```python
from build123d import *

# Parameters (mm, degrees)
SKETCH1_R           = 45
SKETCH1_R_2         = 25
BOSS_EXTRUDE1_DEPTH = 3


with BuildPart() as part:
    # Sketch1 → Boss-Extrude1 (new body)
    with BuildSketch(Plane(origin=(0, 0, 0), x_dir=(1, 0, 0), z_dir=(0, 1, 0))):
        with Locations(Location((0, 0, 0), (0, 0, 270))):
            Circle(SKETCH1_R)
        with Locations(Location((0, 0, 0), (0, 0, 270))):
            Circle(SKETCH1_R_2, mode=Mode.SUBTRACT)
        Polygon((-7.346, 39.573965988), (7.346, 39.573965988), (5.573, 29.223349757), (-5.573, 29.223349757), align=None, mode=Mode.SUBTRACT)
        Polygon((9.785315303, 28.094663273), (13.425160378, 37.945059874), (26.14880561, 30.599059874), (19.438034454, 22.521663273), align=None, mode=Mode.SUBTRACT)
        Polygon((22.521663273, 19.438034454), (30.599059874, 26.14880561), (37.945059874, 13.425160378), (28.094663273, 9.785315303), align=None, mode=Mode.SUBTRACT)
        Polygon((29.223349757, 5.573), (39.573965988, 7.346), (39.573965988, -7.346), (29.223349757, -5.573), align=None, mode=Mode.SUBTRACT)
        Polygon((28.094663273, -9.785315303), (37.945059874, -13.425160378), (30.599059874, -26.14880561), (22.521663273, -19.438034454), align=None, mode=Mode.SUBTRACT)
        Polygon((19.438034454, -22.521663273), (26.14880561, -30.599059874), (13.425160378, -37.945059874), (9.785315303, -28.094663273), align=None, mode=Mode.SUBTRACT)
        Polygon((5.573, -29.223349757), (7.346, -39.573965988), (-7.346, -39.573965988), (-5.573, -29.223349757), align=None, mode=Mode.SUBTRACT)
        Polygon((-9.785315303, -28.094663273), (-13.425160378, -37.945059874), (-26.14880561, -30.599059874), (-19.438034454, -22.521663273), align=None, mode=Mode.SUBTRACT)
        Polygon((-22.521663273, -19.438034454), (-30.599059874, -26.14880561), (-37.945059874, -13.425160378), (-28.094663273, -9.785315303), align=None, mode=Mode.SUBTRACT)
        Polygon((-29.223349757, -5.573), (-39.573965988, -7.346), (-39.573965988, 7.346), (-29.223349757, 5.573), align=None, mode=Mode.SUBTRACT)
        Polygon((-28.094663273, 9.785315303), (-37.945059874, 13.425160378), (-30.599059874, 26.14880561), (-22.521663273, 19.438034454), align=None, mode=Mode.SUBTRACT)
        Polygon((-19.438034454, 22.521663273), (-26.14880561, 30.599059874), (-13.425160378, 37.945059874), (-9.785315303, 28.094663273), align=None, mode=Mode.SUBTRACT)
    extrude(amount=BOSS_EXTRUDE1_DEPTH)


solid = part.part
```
Verification items for the finished model (mm, model axes). Coordinates: 2 decimals unless noted, no trailing zeros. Loops run counter-clockwise (first coordinate to the right, second up) from the corner with the lowest first, then second, coordinate; pieces in that order, holes last. Notation, with made-up numbers: (-0.5, -12.5) - (6.5, -12.5) arc R26 cw to (6.5, 6.5) - close; hole circle Ø3 at (7.25, 62.5). An arc over 180 degrees is marked (long way). Return JSON: item names as keys, results as strings.
1. Thickness scan on L1, parallel to X at y = 1.6, z = 0; L2, parallel to X at y = 1.1, z = -21.5; L3, parallel to Z at x = 25.5, y = 2.5. Record the ranges inside material, lowest first.
Established:
{"L1": "x = -45 to -39.57, -29.22 to -25, 25 to 29.22, 39.57 to 45", "L2": "x = -39.53 to -33.28, -25 to -12.76, 12.76 to 25, 33.28 to 39.53", "L3": "z = -37.08 to -30.97, -29.82 to -21.91, -14.28 to 14.28, 21.91 to 29.82, 30.97 to 37.08"}
2. Section check C-C, the plane y = 2.45. Count the separate pieces of the cut face and the enclosed holes in it, then the cut area to 3 significant figures.
Established:
{"separate pieces": "1", "enclosed holes": "13", "area": "2,790 mm2"}
3. Mould release check, pull along Z, two halves, no side actions. Record for faces 1 (the flat face through (-34.22, 1.48, 19.88)), 2 (the flat face through (24, 3, 10)): +Z half, -Z half, draft (parallel to the pull), parting line (faces both ways), or undercut.
Established:
{"face 1": "undercut", "face 2": "draft"}
4. Go/stop test with flat-tipped pins: pin 1 (1.5 mm diameter, centred on y = 1.5, z = -1.5, fed in from +X); pin 2 (1 mm diameter, centred on x = 25, y = 2, fed in from -Z); pin 3 (0.9 mm diameter, centred on y = 1, z = 2.5, fed in from -X). Record where each tip stops, or that it passes through.
Established:
{"pin 1": "stops at x = 44.99", "pin 2": "stops at z = -37.75", "pin 3": "stops at x = -44.95"}
5. Section check B-B, the plane x = 0. Record the boundary of the cut face in (y, z), then the cut area to 3 significant figures.
Established:
{"outline": "(0, -45) - (3, -45) - (3, -39.57) - (0, -39.57) - close; (0, -29.22) - (3, -29.22) - (3, -25) - (0, -25) - close; (0, 25) - (3, 25) - (3, 29.22) - (0, 29.22) - close; (0, 39.57) - (3, 39.57) - (3, 45) - (0, 45) - close", "area": "57.9 mm2"}
6. Section check A-A, the plane z = 0. Record the boundary of the cut face in (x, y).
Established:
{"outline": "(-45, 0) - (-39.57, 0) - (-39.57, 3) - (-45, 3) - close; (-29.22, 0) - (-25, 0) - (-25, 3) - (-29.22, 3) - close; (25, 0) - (29.22, 0) - (29.22, 3) - (25, 3) - close; (39.57, 0) - (45, 0) - (45, 3) - (39.57, 3) - close"}
